```python
from build123d import *

# Parameters (mm, degrees)
SKIZZE1_R                       = 59
AUFSATZ_LINEAR_AUSTRAGEN1_DEPTH = 6
SKIZZE1_3_R                     = 6
AUFSATZ_LINEAR_AUSTRAGEN2_DEPTH = 2
AUFSATZ_LINEAR_AUSTRAGEN2_TAPER = 30
SKIZZE2_R                       = 4.262826076
SCHNITT_LINEAR_AUSTRAGEN1_DEPTH = 0.5
SCHNITT_LINEAR_AUSTRAGEN1_TAPER = 45


with BuildPart() as part:
    # Skizze1 → Aufsatz-Linear austragen1 (new body)
    with BuildSketch(Plane(origin=(0, 0, 0), x_dir=(1, 0, 0), z_dir=(0, 1, 0))):
        Circle(SKIZZE1_R)
    extrude(amount=AUFSATZ_LINEAR_AUSTRAGEN1_DEPTH)

    # Skizze1_3 → Aufsatz-Linear austragen2 (add)
    with BuildSketch(Plane(origin=(0, 0, 0), x_dir=(1, 0, 0), z_dir=(0, 1, 0))):
        Circle(SKIZZE1_3_R)
    extrude(amount=-AUFSATZ_LINEAR_AUSTRAGEN2_DEPTH, taper=AUFSATZ_LINEAR_AUSTRAGEN2_TAPER)

    # Skizze2 → Schnitt-Linear austragen1 (cut)
    with BuildSketch(Plane.XZ.offset(2)):
        Circle(SKIZZE2_R)
    extrude(amount=-SCHNITT_LINEAR_AUSTRAGEN1_DEPTH, taper=SCHNITT_LINEAR_AUSTRAGEN1_TAPER, mode=Mode.SUBTRACT)


solid = part.part
```
Design review of the part built by this model. Coordinates are the model's own, in mm. Give positions to 0.01 mm unless a question says otherwise; leave off trailing zeros. Loops run counter-clockwise (first coordinate to the right, second up) from the corner with the lowest first, then second, coordinate; pieces in that order, holes last. Notation, with made-up numbers: (-29, -26) -> (18, -26) arc R4 cw to (18, -20) -> close; hole circle Ø1 at (34, 85). An arc over 180 degrees is marked (long way). One line per item, written item: value.
Q1. Draft analysis for pull direction Z (two halves, no side actions). For faces 1 (the cylindrical face through (56.275, 2.958, -17.722)), 2 (the flat face through (-1, 6, -1)), 3 (the flat face through (0, -1.5, 0)), state which applies: pulls with the +Z half, pulls with the -Z half, needs draft (parallel to the pull), parting line crosses it, or undercut.
Numbers:
face 1: parting line crosses it
face 2: needs draft
face 3: undercut
Q2. We need section A-A on x = 0. Give the boundary of the cut face in (y, z).
Numbers:
outline: (-2, -4.85) -> (0, -6) -> (0, -59) -> (6, -59) -> (6, 59) -> (0, 59) -> (0, 6) -> (-2, 4.85) -> (-2, 4.26) -> (-1.5, 3.76) -> (-1.5, -3.76) -> (-2, -4.26) -> close
Q3. We need section D-D on x = 41.5. Give the boundary of the cut face in (y, z).
Numbers:
outline: (0, -41.94) -> (6, -41.94) -> (6, 41.94) -> (0, 41.94) -> close
Q4. We need section C-C on z = 16. Give the boundary of the cut face in (x, y), and give its area (3 significant figures).
Numbers:
outline: (-56.79, 0) -> (56.79, 0) -> (56.79, 6) -> (-56.79, 6) -> close
area: 681 mm^2
Q5. For pin 1 Ø4 at (x, y) = (-23, 0) entering from +Z; pin 2 Ø4 at (x, y) = (31.5, 0.5) entering from -Z; pin 3 Ø2.5 at (x, z) = (0, 0) entering from -Y, all flat-tipped, find the tip position at first contact; note any pin that passes through.
Numbers:
pin 1: stops at z = 55.14
pin 2: stops at z = -51.1
pin 3: stops at y = -1.5
Q6. We need section B-B on y = 3. Give the boundary of the cut face in (x, z).
Numbers:
outline: circle Ø118 at (0, 0)
Q7. For L1, parallel to Y at x = 28, z = 13; L2, parallel to Z at x = -50, y = 0.25; L3, parallel to X at y = 4, z = 2, list the stretches that pass through material, from the lowest coordinate up.
Numbers:
L1: y = 0 to 6
L2: z = -31.32 to 31.32
L3: x = -58.97 to 58.97
